Input: part model. Units: mm. Frame: model coordinates. A direction names the side the tool comes from. Round coordinates to 2 decimals unless told otherwise and drop trailing zeros. Loops run counter-clockwise (first coordinate to the right, second up) from the corner with the lowest first, then second, coordinate; pieces in that order, holes last. Notation, with made-up numbers: (-13.5, 37.25) -> (43.5, 37.25) arc R21 cw to (43.5, 58.25) -> close; hole circle Ø6 at (2, -16). An arc over 180 degrees is marked (long way). Answer in a Markdown table with one row per item. Add a question column.
Q1. Reachability of faces 1 (the face through (-27.5, 14, -18)), 2 (the face through (-27.5, 69, 0)), 3 (the face through (0, 14, -3)), 4 (the face through (-45.5, 45, 0)), 5 (the face through (70, 12, 0)) from +Z, -Z, +X, -X, +Y, -Y: full face, straight path, thin tool, end or side. Return the list, or none.
Q2. Pin query (flat end, axial travel): pin 1 (8.5 mm diameter, centred on y = 13.5, z = 16, fed in from +X); pin 2 (15 mm diameter, centred on x = 6, z = 4, fed in from +Y); pin 3 (8.5 mm diameter, centred on x = -6.5, z = 12.5, fed in from -Y). Return the tip coordinate at first contact, or that it passes through.
Q3. Mould query, pull axis Z, two halves, no side actions, for faces 6 (the face through (27.5, 69, 0)), 7 (the face through (-6, 38, 25)), 8 (the face through (36.626, 65.932, 1.041)). Classes: pulls with the +Z half, pulls with the -Z half, needs draft (parallel to the pull), parting line crosses it, or undercut.
Q4. Section B-B, the plane x = 77.5. Output: boundary loops of the cut face in (y, z), and give its area (3 significant figures).
Q5. Ray query, L1, parallel to X at y = 7, z = -7; L2, parallel to X at y = 57, z = 12.5; L3, parallel to Y at x = 38.25, z = 0. Return the intervals inside material, ascending. Write a range as from..to.
Q6. Section A-A, the plane y = 58. Output: boundary loops of the cut face in (x, z), and give its area (3 significant figures).
Q7. Section C-C, the plane y = 85. Output: boundary loops of the cut face in (x, z).
Q8. Section D-D, the plane x = -25.5. Output: boundary loops of the cut face in (y, z).
```python
from build123d import *

# Parameters (mm, degrees)
SKETCH1_R           = 7.5
BOSS_EXTRUDE1_DEPTH = 98
SKETCH2_W           = 49.5
SKETCH2_H           = 86
SKETCH2_W_2         = 55
SKETCH2_H_2         = 58
CUT_EXTRUDE1_DEPTH  = 51
SKETCH3_W           = 55
SKETCH3_H           = 28
CUT_EXTRUDE2_DEPTH  = 51
SKETCH4_W           = 55
SKETCH4_H           = 8
BOSS_EXTRUDE2_DEPTH = 28
SKETCH5_R           = 8
CUT_EXTRUDE3_DEPTH  = 141.5


with BuildPart() as part:
    # Sketch1 → Boss-Extrude1 (new body)
    with BuildSketch(Plane(origin=(0, 0, 0), x_dir=(1, 0, 0), z_dir=(0, 1, 0))):
        Polygon((-95, 25), (-95, -5), (-70, -25), (70, -25), (95, -5), (95, 25), align=None)
        with Locations((-77.5, 7)):
            Circle(SKETCH1_R, mode=Mode.SUBTRACT)
        with Locations((77.5, 7)):
            Circle(SKETCH1_R, mode=Mode.SUBTRACT)
    extrude(amount=BOSS_EXTRUDE1_DEPTH)

    # Sketch2 → Cut-Extrude1 (cut, through all)
    with BuildSketch(Plane.XY.offset(25)):
        with Locations((-70.25, 55)):
            Rectangle(SKETCH2_W, SKETCH2_H)
        with Locations((70.25, 55)):
            Rectangle(SKETCH2_W, SKETCH2_H)
        with Locations((0, 69)):
            Rectangle(SKETCH2_W_2, SKETCH2_H_2)
    extrude(amount=-CUT_EXTRUDE1_DEPTH, mode=Mode.SUBTRACT)

    # Sketch3 → Cut-Extrude2 (cut, through all)
    with BuildSketch(Plane.XY.offset(25)):
        with Locations((0, 14)):
            Rectangle(SKETCH3_W, SKETCH3_H)
    extrude(amount=-CUT_EXTRUDE2_DEPTH, mode=Mode.SUBTRACT)

    # Sketch4 → Boss-Extrude2 (add)
    with BuildSketch(Plane.XZ.offset(-28)):
        with Locations((0, -7)):
            Rectangle(SKETCH4_W, SKETCH4_H)
    extrude(amount=BOSS_EXTRUDE2_DEPTH)

    # Sketch5 → Cut-Extrude3 (cut, through all)
    with BuildSketch(Plane(origin=(45.5, 0, 0), x_dir=(0, 0, -1), z_dir=(1, 0, 0))):
        with BuildLine():
            ThreePointArc((2.26e-07, 98), (13.247648961, 95.742546244), (25, 89.224989992))
            Line((25, 89.224989992), (25, 98))
            Line((25, 98), (2.26e-07, 98))
        make_face()
        with BuildLine():
            ThreePointArc((-25, 89.224989992), (-13.247648747, 95.742546319), (2.26e-07, 98))
            Line((2.26e-07, 98), (-25, 98))
            Line((-25, 98), (-25, 89.224989992))
        make_face()
        with Locations((0, 58)):
            Circle(SKETCH5_R)
    extrude(amount=-CUT_EXTRUDE3_DEPTH, mode=Mode.SUBTRACT)


solid = part.part
```
Answer block:
| question | item | result |
|---|---|---|
| 1 | face 1 | -Z, -Y |
| 1 | face 2 | +Z, -Z, +Y |
| 1 | face 3 | +Z, -Y |
| 1 | face 4 | +Z, -Z, -X, +Y |
| 1 | face 5 | +Z, -Z, +X, +Y |
| 2 | pin 1 | x = 86.22 |
| 2 | pin 2 | y = 40 |
| 2 | pin 3 | y = 28 |
| 3 | face 6 | needs draft |
| 3 | face 7 | pulls with the +Z half |
| 3 | face 8 | undercut |
| 4 | outline | (0, -25) -> (12, -25) -> (12, -14.5) -> (0, -14.5) -> close; (0, 0.5) -> (12, 0.5) -> (12, 19) -> (0, 19) -> close |
| 4 | area | 348 mm^2 |
| 5 | L1 | -95..-85, -70..70, 85..95 |
| 5 | L2 | -45.5..-27.5, 27.5..45.5 |
| 5 | L3 | 0..50, 66..98 |
| 6 | outline | (-45.5, -25) -> (-27.5, -25) -> (-27.5, -8) -> (-45.5, -8) -> close; (-45.5, 8) -> (-27.5, 8) -> (-27.5, 25) -> (-45.5, 25) -> close; (27.5, -25) -> (45.5, -25) -> (45.5, -8) -> (27.5, -8) -> close; (27.5, 8) -> (45.5, 8) -> (45.5, 25) -> (27.5, 25) -> close |
| 6 | area | 1,220 mm^2 |
| 7 | outline | (-45.5, -25) -> (-27.5, -25) -> (-27.5, 25) -> (-45.5, 25) -> close; (27.5, -25) -> (45.5, -25) -> (45.5, 25) -> (27.5, 25) -> close |
| 8 | outline | (0, -11) -> (28, -11) -> (28, -25) -> (40, -25) -> (40, 25) -> (28, 25) -> (28, -3) -> (0, -3) -> close |
